Job drawing, mm, ordinate dimensions from the low corner. One solid piece. Give positions to 0.01 mm unless a question says otherwise; leave off trailing zeros. Loops run counter-clockwise (first coordinate to the right, second up) from the corner with the lowest first, then second, coordinate; pieces in that order, holes last. Notation, with made-up numbers: (35.5, 15) - (61.5, 15) arc R21 ccw to (61.5, 30) - close; hole circle Ø6 at (75.5, 81.25). An arc over 180 degrees is marked (long way). Use a Markdown table: item, result.
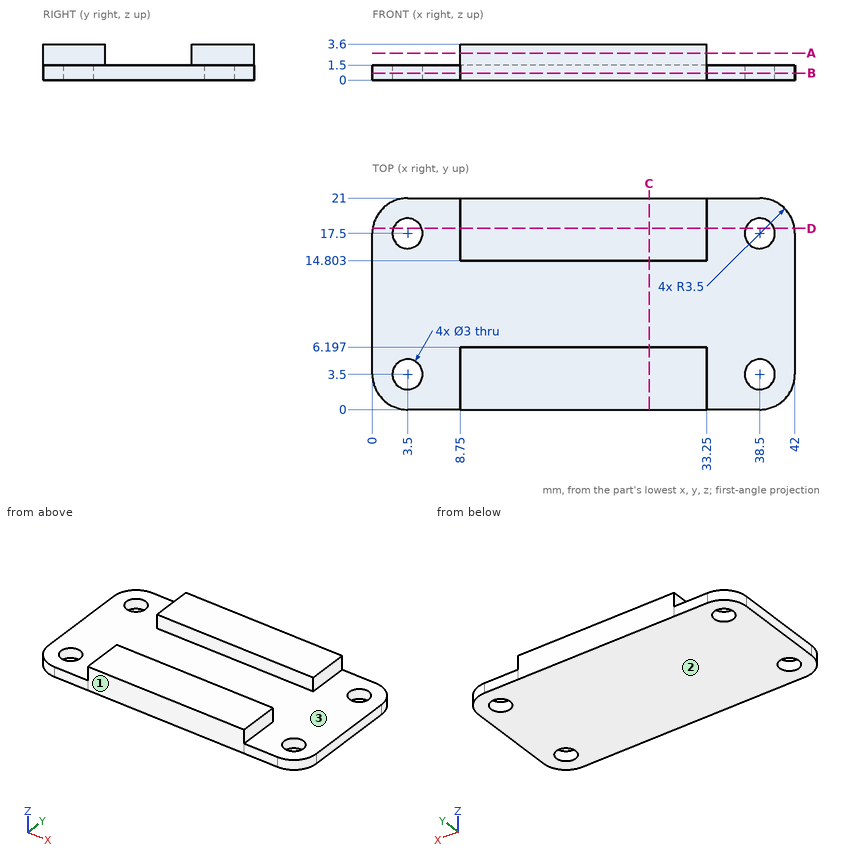
(1) Drill centre lines: probe 1 along Y at (x, z) = (11, 3.45); probe 2 along X at (y, z) = (18.25, 1.2); probe 3 along Z at (x, y) = (17, 11.25). Where is each one in solid material? Low to high. Write a range as [from, to].
Computed:
| item | result |
|---|---|
| probe 1 | [0, 6.2], [14.8, 21] |
| probe 2 | [0.08, 2.2], [4.8, 37.2], [39.8, 41.92] |
| probe 3 | [0, 1.5] |
(2) Mould opens along Y. For the marked faces 1, 2 and 3 say: pulls with the +Y half, pulls with the -Y half, needs draft (parallel to the pull), parting line crosses it, or undercut.
Computed:
| item | result |
|---|---|
| face 1 | pulls with the -Y half |
| face 2 | needs draft |
| face 3 | undercut |
(3) Slice it at C-C, the plane x = 27.5. Write the cut outline in (y, z).
Computed:
| item | result |
|---|---|
| outline | (0, 0) - (21, 0) - (21, 3.6) - (14.8, 3.6) - (14.8, 1.5) - (6.2, 1.5) - (6.2, 3.6) - (0, 3.6) - close |
(4) Slice it at D-D, the plane y = 18. Count the separate pieces of the cut face and the enclosed holes in it, plus the area to 3 significant figures.
Computed:
| item | result |
|---|---|
| separate pieces | 3 |
| enclosed holes | 0 |
| area | 106 mm² |
(5) Pin check, flat tips, straight feed: P1, Ø5, axis at x = 3.5, y = 17.5, coming from the +Z side; P2, Ø1.8, axis at x = 3.5, y = 3.5, coming from the +Z side; P3, Ø1.8, axis at y = 2, z = 1, coming from the -X side. Stop position of each tip, or through.
Computed:
| item | result |
|---|---|
| P1 | z = 1.5 |
| P2 | through |
| P3 | x = 0.05 |
(6) Slice it at A-A, the plane z = 2.7. Write the cut outline in (x, y), plus the area to 3 significant figures.
Computed:
| item | result |
|---|---|
| outline | (8.75, 0) - (33.25, 0) - (33.25, 6.2) - (8.75, 6.2) - close; (8.75, 14.8) - (33.25, 14.8) - (33.25, 21) - (8.75, 21) - close |
| area | 304 mm² |
(7) Slice it at B-B, the plane z = 0.7. Write the cut outline in (x, y).
Computed:
| item | result |
|---|---|
| outline | (0, 3.5) arc R3.5 ccw to (3.5, 0) - (38.5, 0) arc R3.5 ccw to (42, 3.5) - (42, 17.5) arc R3.5 ccw to (38.5, 21) - (3.5, 21) arc R3.5 ccw to (0, 17.5) - close; hole circle Ø3 at (3.5, 3.5); hole circle Ø3 at (3.5, 17.5); hole circle Ø3 at (38.5, 3.5); hole circle Ø3 at (38.5, 17.5) |
